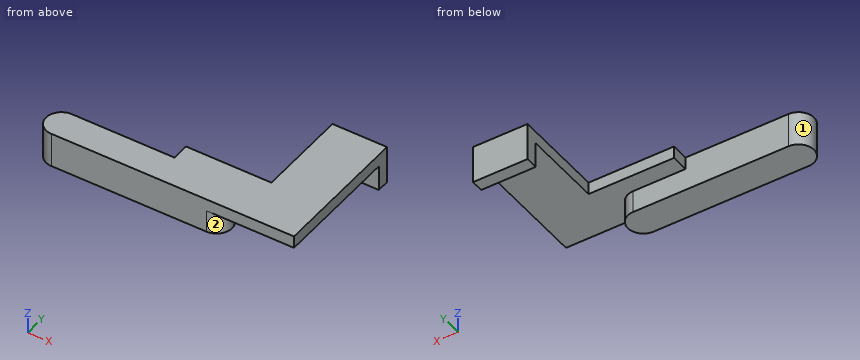
from build123d import *

# Parameters (mm, degrees)
F1_DEPTH = 4.6482
F2_W     = 11.2398419182
F2_H     = 2.54
F3_DEPTH = 2.54
F4_DEPTH = 5.2832


with BuildPart() as f1:
    # F0 (on Top) → F1 (new body)
    with BuildSketch(Plane.XY):
        with BuildLine():
            ThreePointArc((0, 6.35), (-3.175, 3.175), (0, 0))
            Line((0, 0), (31.9786, 0))
            ThreePointArc((31.9786, 0), (35.1536, 3.175), (31.9786, 6.35))
            Line((31.9786, 6.35), (0, 6.35))
        make_face()
    extrude(amount=F1_DEPTH)

    # F2 (on face) → F3 (join)
    with BuildSketch(Plane.XY.offset(4.6482)):
        Polygon((38.7858, 9.9314), (38.7858, 0), (50.0256419182, 0), (50.0256419182, 26.3525), (38.7858, 26.3525), align=None)
        with BuildLine():
            Line((31.9786, 0), (35.1536, 0))
            Line((35.1536, 0), (38.7858, 0))
            Line((38.7858, 0), (38.7858, 9.9314))
            Line((38.7858, 9.9314), (35.1536, 9.9314))
            Line((35.1536, 9.9314), (21.18106, 9.9314))
            Line((21.18106, 9.9314), (21.18106, 6.35))
            Line((21.18106, 6.35), (31.9786, 6.35))
            ThreePointArc((31.9786, 6.35), (35.1536, 3.175), (31.9786, 0))
        make_face()
        with BuildLine():
            Line((21.18106, 0), (31.9786, 0))
            ThreePointArc((31.9786, 0), (35.1536, 3.175), (31.9786, 6.35))
            Line((31.9786, 6.35), (21.18106, 6.35))
            Line((21.18106, 6.35), (21.18106, 0))
        make_face()
        with Locations((44.4057209591, 27.6225)):
            Rectangle(F2_W, F2_H)
        with BuildLine():
            Line((0, 0), (21.18106, 0))
            Line((21.18106, 0), (21.18106, 6.35))
            Line((21.18106, 6.35), (0, 6.35))
            ThreePointArc((0, 6.35), (-3.175, 3.175), (0, 0))
        make_face()
    extrude(amount=F3_DEPTH)

    # F2 (on face) → F4 (join)
    with BuildSketch(Plane.XY.offset(4.6482)):
        with Locations((44.4057209591, 27.6225)):
            Rectangle(F2_W, F2_H)
    extrude(amount=-F4_DEPTH)


solid = f1.part
Work out the finished part from the listing and answer in its coordinate system (mm). Face numbers are marked on the shaded views. A direction names the side the tool comes from. Coordinates: 2 decimals unless noted, no trailing zeros. Loops run counter-clockwise (first coordinate to the right, second up) from the corner with the lowest first, then second, coordinate; pieces in that order, holes last. Notation, with made-up numbers: M -19.75,-17.75 L 9.25,-17.75 A14 ccw 9.25,-0.75 Z; hole C -34.5,46.5 d11. An arc over 180 degrees is marked long. Answer in a Markdown table with one row per item. Add a question column.
1. Find section C-C, the plane x = 24. Write down the section's boundary in (y, z), then the cut area to 3 significant figures.
2. Consider L1, parallel to Y at x = 10.5, z = 3.75; L2, parallel to Y at x = 41, z = 1.75; L3, parallel to X at y = 7.25, z = 5.25. Determine where each line is inside the solid, lowest interval first.
3. Flat-ended cylindrical pins translate along their axes: P1, Ø3, axis at y = 7.5, z = 6.5, coming from the -X side; P2, Ø10, axis at x = 4.5, y = 5, coming from the -Z side; P3, Ø2, axis at x = 29.5, z = 6.5, coming from the +Y side. Find the tip coordinate at first contact, or state that the pin passes through.
4. Find section D-D, the plane y = 22. Write down the section's boundary in (x, z), then the cut area to 3 significant figures.
5. A tool of negligible diameter and unlimited length cuts with its end or side. For the marked faces 1 and 2, from which of +Z, -Z, +X, -X, +Y, -Y can it reach the whole face along a straight path? Write none if from no direction.
Reported:
| question | item | result |
|---|---|---|
| 1 | outline | M 0,0 L 6.35,0 L 6.35,4.65 L 9.93,4.65 L 9.93,7.19 L 0,7.19 Z |
| 1 | area | 54.7 mm^2 |
| 2 | L1 | y = 0 to 6.35 |
| 2 | L2 | y = 26.35 to 28.89 |
| 2 | L3 | x = 21.18 to 50.03 |
| 3 | P1 | stops at x = -1.45 |
| 3 | P2 | stops at z = 0 |
| 3 | P3 | stops at y = 9.93 |
| 4 | outline | M 38.79,4.65 L 50.03,4.65 L 50.03,7.19 L 38.79,7.19 Z |
| 4 | area | 28.5 mm^2 |
| 5 | face 1 | +Z, -Z, -X |
| 5 | face 2 | -Z, +X |
